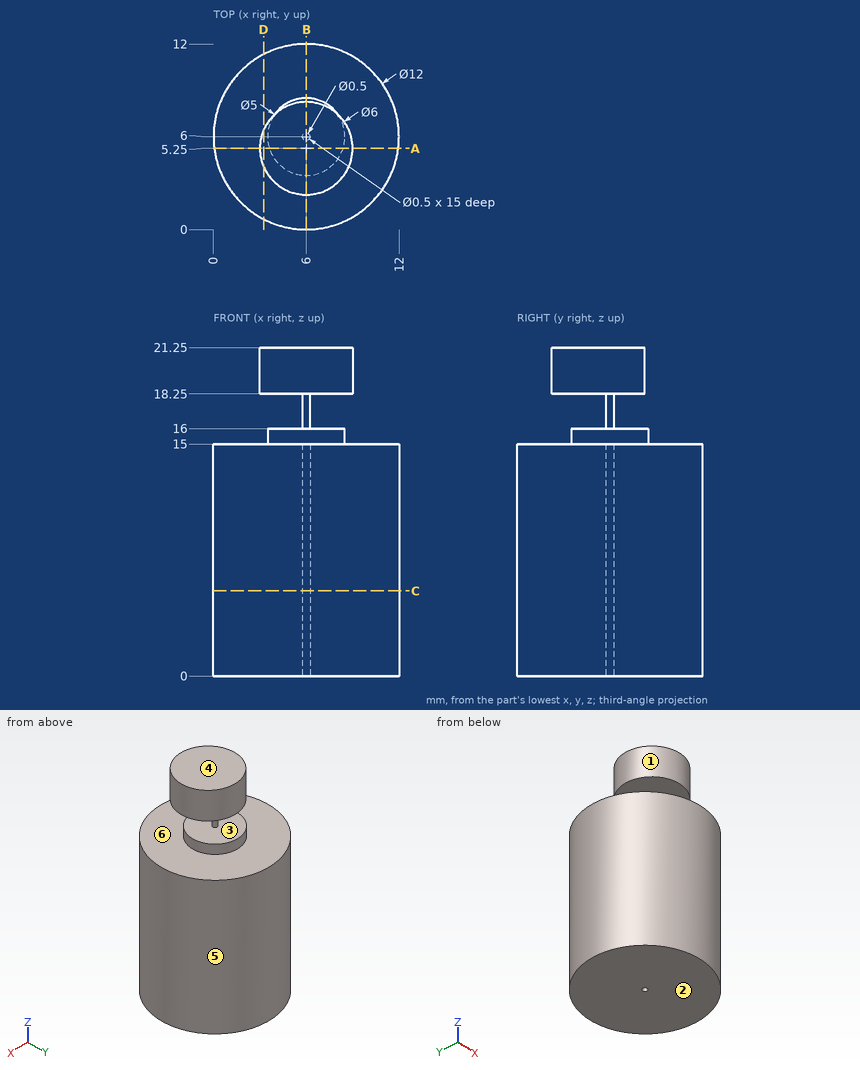
Source: three-view drawing plus pictorial views. Frame: mm from the lowest corner of the part. A direction names the side the tool comes from. Give positions to 0.01 mm unless a question says otherwise; leave off trailing zeros. Write each loop counter-clockwise with the first axis right and the second up, starting at its lowest first coordinate (ties: lowest second). Pieces come first, ordered by that corner, then holes. Notation, with made-up numbers: (56.5, 27.5) -> (77.5, 27.5) arc R29 cw to (77.5, 48.5) -> close; hole circle Ø2 at (38.25, -9.75). An arc over 180 degrees is marked (long way). Write item = value, one per line.
Q1. Cut plane C-C on z = 5.5. Return loops of the section in (x, y), then the cut area to 3 significant figures.
Here are the results:
outline = circle Ø12 at (6, 6); hole circle Ø0.5 at (6, 6)
area = 113 mm²
Q2. Mould query, pull axis Z, two halves, no side actions, for the marked faces 1, 2, 3 and 4. Classes: +Z half, -Z half, draft (parallel to the pull), parting line (faces both ways), or undercut.
Here are the results:
face_1 = draft
face_2 = -Z half
face_3 = undercut
face_4 = +Z half
Q3. Line query: line 1 (Y direction, x = 6, z = 3.5); line 2 (Z direction, x = 8, y = 6); line 3 (Z direction, x = 6.5, y = 1). Output: solid intervals per line, ascending. Write a range as from..to.
Here are the results:
line_1 = 0..5.75, 6.25..12
line_2 = 0..16, 18.25..21.25
line_3 = 0..15
Q4. First-contact query: pin 1 (2 mm diameter, centred on x = 2, z = 3.5, fed in from -Y); pin 2 (1 mm diameter, centred on x = 7.5, z = 11, fed in from +Y); pin 3 (6 mm diameter, centred on y = 2, z = 12.5, fed in from -X). Flat tips, straight axial feed; report the tip coordinate or a pass-through.
Here are the results:
pin_1 = 0.8
pin_2 = 11.92
pin_3 = 0.08
Q5. Reachability of the marked faces 5 and 6 from +Z, -Z, +X, -X, +Y, -Y: full face, straight path, thin tool, end or side. Return the list, or none.
Here are the results:
face_5 = +Z, -Z
face_6 = none
Q6. Cut plane B-B on x = 6. Return loops of the section in (y, z).
Here are the results:
outline = (0, 0) -> (5.75, 0) -> (5.75, 15) -> (6.25, 15) -> (6.25, 0) -> (12, 0) -> (12, 15) -> (8.5, 15) -> (8.5, 16) -> (6.25, 16) -> (6.25, 18.25) -> (8.25, 18.25) -> (8.25, 21.25) -> (2.25, 21.25) -> (2.25, 18.25) -> (5.75, 18.25) -> (5.75, 16) -> (3.5, 16) -> (3.5, 15) -> (0, 15) -> close
Q7. Cut plane A-A on y = 5.25. Return loops of the section in (x, z).
Here are the results:
outline = (0.05, 0) -> (11.95, 0) -> (11.95, 15) -> (8.38, 15) -> (8.38, 16) -> (3.62, 16) -> (3.62, 15) -> (0.05, 15) -> close; (3, 18.25) -> (9, 18.25) -> (9, 21.25) -> (3, 21.25) -> close
Q8. Cut plane D-D on x = 3.25. Return loops of the section in (y, z), then the cut area to 3 significant figures.
Here are the results:
outline = (0.67, 0) -> (11.33, 0) -> (11.33, 15) -> (0.67, 15) -> close; (4.05, 18.25) -> (6.45, 18.25) -> (6.45, 21.25) -> (4.05, 21.25) -> close
area = 167 mm²
